from build123d import *

# Parameters (mm, degrees)
SKETCH_1_R          = 4
EXTRUDE_1_DEPTH     = 6.5
SKETCH_3_R          = 6.5
EXTRUDE_2_DEPTH     = 12
SKETCH_2_R          = 2.4
CUT_EXTRUDE_1_DEPTH = 16
CUT_EXTRUDE_START   = -12
SKETCH_4_R          = 4
CUT_EXTRUDE_2_DEPTH = 12


with BuildPart() as part:
    # 草图1 → 凸台-拉伸1 (new, symmetric)
    with BuildSketch(Plane(origin=(0, 0, 0), x_dir=(1, 0, 0), z_dir=(0, 1, 0))):
        with BuildLine():
            Line((-15, 3), (-9.464557528, 19.228335609))
            ThreePointArc((-9.464557528, 19.228335609), (0, 26), (9.464557528, 19.228335609))
            Line((9.464557528, 19.228335609), (15, 3))
            Line((15, 3), (27.5, 3))
            Line((27.5, 3), (27.5, -3))
            Line((27.5, -3), (-27.5, -3))
            Line((-27.5, -3), (-27.5, 3))
            Line((-27.5, 3), (-15, 3))
        make_face()
        with Locations(Location((0, 16, 0), (0, 0, 90))):
            Circle(SKETCH_1_R, mode=Mode.SUBTRACT)
    extrude(amount=EXTRUDE_1_DEPTH, both=True)

    # 草图3 → 凸台-拉伸2 (add)
    with BuildSketch(Plane(origin=(0, 3.5, 0), x_dir=(1, 0, 0), z_dir=(0, 1, 0))):
        with Locations(Location((0, 16, 0), (0, 0, 270))):
            Circle(SKETCH_3_R)
    extrude(amount=-EXTRUDE_2_DEPTH)

    # 草图2 → 切除-拉伸1 (cut)
    with BuildSketch(Plane(origin=(0, 0, -3), x_dir=(-1, 0, 0), z_dir=(0, 0, -1))):
        with Locations((20.5, 0)):
            Circle(SKETCH_2_R)
        with Locations((-20.5, 0)):
            Circle(SKETCH_2_R)
    extrude(amount=-CUT_EXTRUDE_1_DEPTH, mode=Mode.SUBTRACT)

    # 草图4 → 切除-拉伸2 (cut)
    with BuildSketch(Plane(origin=(0, 3.5, 0), x_dir=(1, 0, 0), z_dir=(0, 1, 0)).offset(CUT_EXTRUDE_START)):
        with Locations(Location((0, 16, 0), (0, 0, 90))):
            Circle(SKETCH_4_R)
    extrude(amount=CUT_EXTRUDE_2_DEPTH, mode=Mode.SUBTRACT)


solid = part.part
CAD build for the part. Positions are in the model's coordinates, mm. A direction names the side the tool comes from. Give positions to 0.01 mm unless a question says otherwise; leave off trailing zeros. Loops run counter-clockwise (first coordinate to the right, second up) from the corner with the lowest first, then second, coordinate; pieces in that order, holes last. Notation, with made-up numbers: M 67.25,74.25 L 124.25,74.25 A17 ccw 124.25,107.25 Z; hole C 63.5,37 d5. An arc over 180 degrees is marked long. One line per question, with ' | ' between items. Start each with the question number.
1. Two-plate mould, pull along X, no slides. Class faces 1 (the face through (0, 6.5, -8)), 2 (the face through (-12.27, 0.09, -11)), 3 (the face through (0, -1, -12)): pulls with the +X half, pulls with the -X half, needs draft (parallel to the pull), parting line crosses it, or undercut.
2. Saw through at A-A on x = 20.5. Give the cut face in (y, z).
3. Probe L1, parallel to Y at x = 20.5, z = 0; L2, parallel to X at y = 1, z = 1.75; L3, parallel to Z at x = -22, y = -4.75. List the from-to ranges inside material, lowest first. Write a range as from..to.
4. Saw through at D-D on x = 0. Give the cut face in (y, z), plus the area to 3 significant figures.
5. 3-axis set-ups, long thin cutter, end or side, ignore diameter. For faces 4 (the face through (-23, 2, -3)), 5 (the face through (23, 2, -3)), 6 (the face through (0.286, -7.486, -22.494)): which of +Z, -Z, +X, -X, +Y, -Y reach the whole face in a straight line?
6. Saw through at C-C on y = -0.75. Give the cut face in (x, z), plus the area to 3 significant figures.
7. Saw through at B-B on z = -18. Give the cut face in (x, y).
8. Flat gauge pins, fed straight in: pin 1 (1.5 mm diameter, centred on y = 0.5, z = -22.5, fed in from -X); pin 2 (6 mm diameter, centred on y = -2, z = -15, fed in from -X); pin 3 (6.5 mm diameter, centred on x = 0, z = -16, fed in from +Y); pin 4 (8.5 mm diameter, centred on x = 5.5, z = -5, fed in from -Y). Where does each tip first touch, or does it go through?
Result sheet:
1) face 1: needs draft | face 2: pulls with the -X half | face 3: undercut
2) outline: M -6.5,-3 L -2.4,-3 L -2.4,3 L -6.5,3 Z; M 2.4,-3 L 6.5,-3 L 6.5,3 L 2.4,3 Z
3) L1: y = -6.5..-2.4, 2.4..6.5 | L2: x = -27.5..-22.68, -18.32..18.32, 22.68..27.5 | L3: z = -3..3
4) outline: M -8.5,-22.5 L -6.5,-22.5 L -6.5,-26 L 6.5,-26 L 6.5,-20 L -8.5,-20 Z; M -8.5,-12 L 6.5,-12 L 6.5,3 L -6.5,3 L -6.5,-9.5 L -8.5,-9.5 Z | area: 283 mm^2
5) face 4: -Z, -X, +Y, -Y | face 5: -Z, +X, +Y, -Y | face 6: -Y
6) outline: M -27.5,-3 L -22.78,-3 L -22.78,3 L -27.5,3 Z; M -18.22,-3 L -15,-3 L -9.46,-19.23 A10 ccw 9.46,-19.23 L 15,-3 L 18.22,-3 L 18.22,3 L -18.22,3 Z; M 22.78,-3 L 27.5,-3 L 27.5,3 L 22.78,3 Z; hole C 0,-16 d8 | area: 716 mm^2
7) outline: M -9.88,-6.5 L -6.18,-6.5 L -6.18,-8.5 L -3.46,-8.5 L -3.46,6.5 L -9.88,6.5 Z; M 3.46,-8.5 L 6.18,-8.5 L 6.18,-6.5 L 9.88,-6.5 L 9.88,6.5 L 3.46,6.5 Z
8) pin 1: stops at x = -8.18 | pin 2: stops at x = -11.93 | pin 3: passes through | pin 4: stops at y = -6.5
